```python
from build123d import *

# Parameters (mm, degrees)
F1_DEPTH  = 6.35
F2_W      = 19.05
F2_H      = 50.8
F2_R      = 3.4537028987
F3_DEPTH  = 6.35
F4_W      = 19.05
F4_H      = 9.525
F5_DEPTH  = 12.7
F6_R      = 2.54
F7_R      = 3.4537028987
F8_DEPTH  = 3.175
F9_R      = 5.08
F10_SIZE  = 5.08
F11_R     = 2.54
F12_R     = 0.79375
F13_DEPTH = 25.4


with BuildPart() as f1:
    # F0 (on Front) → F1 (new body)
    with BuildSketch(Plane.XZ):
        Polygon((38.1, 57.15), (-38.1, 57.15), (-38.1, 44.45), (-9.525, 44.45), (-9.525, 0), (0, 0), (9.525, 0), (9.525, 44.45), (38.1, 44.45), align=None)
    extrude(amount=F1_DEPTH)

    # F2 (on face) → F3 (join)
    with BuildSketch(Plane(origin=(0, 0, 0), x_dir=(1, 0, 0), z_dir=(0, 0, -1))):
        with Locations((0, 25.4)):
            Rectangle(F2_W, F2_H)
        with Locations((0, 43.1535504758)):
            Circle(F2_R, mode=Mode.SUBTRACT)
    extrude(amount=F3_DEPTH)

    # F4 (on face) → F5 (join)
    with BuildSketch(Plane.XZ.offset(6.35)):
        with Locations((0, 4.7625)):
            Rectangle(F4_W, F4_H)
    extrude(amount=F5_DEPTH)

    # F6
    f6_edges = [f1.edges().sort_by_distance(p)[0] for p in [
        (0, -19.05, 9.525),
        (0, -19.05, 0),
    ]]
    fillet(f6_edges, radius=F6_R)

    # F7 (on face) → F8 (cut)
    with BuildSketch(Plane.XY):
        Polygon((-6.5624518347, -43.1535504758), (-3.2812259174, -48.8368004758), (3.2812259174, -48.8368004758), (6.5624518347, -43.1535504758), (3.2812259174, -37.4703004758), (-3.2812259174, -37.4703004758), align=None)
        with Locations((0, -43.1535504758)):
            Circle(F7_R, mode=Mode.SUBTRACT)
    extrude(amount=-F8_DEPTH, mode=Mode.SUBTRACT)

    # F9
    f9_edges = [f1.edges().sort_by_distance(p)[0] for p in [
        (-9.525, -3.175, 44.45),
        (9.525, -3.175, 44.45),
    ]]
    fillet(f9_edges, radius=F9_R)

    # F10
    f10_edges = [f1.edges().sort_by_distance(p)[0] for p in [
        (0, -6.35, 57.15),
        (-26.3525, -6.35, 44.45),
        (11.012898, -6.35, 42.962102),
    ]]
    chamfer(f10_edges, length=F10_SIZE)

    # F11
    f11_edges = [f1.edges().sort_by_distance(p)[0] for p in [
        (-6.985, -3.81, 9.525),
        (6.985, -3.81, 9.525),
        (0, -6.35, 9.525),
    ]]
    fillet(f11_edges, radius=F11_R)

    # F12 (on face) → F13 (cut)
    with BuildSketch(Plane.XY.offset(57.15)):
        with Locations((34.925, 0)):
            Circle(F12_R)
        with Locations((-34.925, 0)):
            Circle(F12_R)
    extrude(amount=-F13_DEPTH, mode=Mode.SUBTRACT)


solid = f1.part
```
Geometry check sheet. Reference: the model listing, model coordinates, mm. A direction names the side the tool comes from. Give positions to 0.01 mm unless a question says otherwise; leave off trailing zeros. Order: outer loops, then holes, each group sorted by start corner. A loop starts at its lowest first (then second) coordinate and runs counter-clockwise, first axis right, second up.
1. Thickness scan on L1, parallel to Y at x = 0, z = -4; L2, parallel to Y at x = -24, z = 51.5. Record the ranges inside material, lowest first.
2. Section check D-D, the plane x = 31. Enter the section's corners in (y, z).
3. Section check C-C, the plane y = -34.5. Enter the section's corners in (x, z) (3 decimals).
4. Section check B-B, the plane z = 18.5. Enter the section's corners in (x, y) (3 decimals).
5. Release check for a two-part mould opening along X. For faces 1 (the face through (-4.94, -45.96, -1.57)), 2 (the face through (0, 0, 33)), 3 (the face through (9.59, -3.21, 44.28)), 4 (the face through (3, -41, -3.175)) record: pulls with the +X half, pulls with the -X half, needs draft (parallel to the pull), parting line crosses it, or undercut.
6. Section check A-A, the plane x = 0. Enter the section's corners in (y, z) (3 decimals).
7. Gauge pin test, flat ends, axial feed: pin 1 Ø5.5 at (x, y) = (0, -39) entering from +Z; pin 2 Ø2.5 at (x, z) = (1, -1.5) entering from +Y; pin 3 Ø0.6 at (x, y) = (28, -0.5) entering from -Z; pin 4 Ø10 at (y, z) = (-9, 0.5) entering from +X (3 decimals). Record the tip position at first contact, or that the pin passes through.
8. Access from +Z, -Z, +X, -X, +Y, -Y to the whole of each face (thin tool, end or side, straight path). Record for faces 5 (the face through (-26.52, -3.77, 46.95)), 6 (the face through (9.525, -18, 1)), 7 (the face through (-9.7, -3.21, 44.39)).
Values follow:
1. L1: y = -50.8 to -46.61, -39.7 to 0
1. L2: y = -6.35 to 0
2. outline: (-6.35, 49.53) - (-1.27, 44.45) - (0, 44.45) - (0, 57.15) - (-1.27, 57.15) - (-6.35, 52.07) - close
3. outline: (-9.525, -6.35) - (9.525, -6.35) - (9.525, 0) - (-9.525, 0) - close
4. outline: (-9.525, -1.27) - (-4.445, -6.35) - (4.445, -6.35) - (9.525, -1.27) - (9.525, 0) - (-9.525, 0) - close
5. face 1: undercut
5. face 2: needs draft
5. face 3: pulls with the +X half
5. face 4: undercut
6. outline: (-50.8, -6.35) - (-46.607, -6.35) - (-46.607, -3.175) - (-48.837, -3.175) - (-48.837, 0) - (-50.8, 0) - close; (-39.7, -6.35) - (0, -6.35) - (0, 57.15) - (-1.27, 57.15) - (-6.35, 52.07) - (-6.35, 12.065) arc R2.54 cw to (-8.89, 9.525) - (-16.51, 9.525) arc R2.54 ccw to (-19.05, 6.985) - (-19.05, 2.54) arc R2.54 cw to (-21.59, 0) - (-37.47, 0) - (-37.47, -3.175) - (-39.7, -3.175) - close
7. pin 1: stops at z = 0
7. pin 2: stops at y = 0
7. pin 3: stops at z = 44.45
7. pin 4: stops at x = 9.525
8. face 5: -Z, -X, -Y
8. face 6: -Z, +X, +Y, -Y
8. face 7: -X, -Y
